Could you check a few things on this model? Use its own coordinates, in mm. Face numbers are marked on the shaded views. A direction names the side the tool comes from. Round coordinates to 2 decimals unless told otherwise and drop trailing zeros. Loops run counter-clockwise (first coordinate to the right, second up) from the corner with the lowest first, then second, coordinate; pieces in that order, holes last. Notation, with made-up numbers: (-26, -19) -> (-2, -19) arc R18 cw to (-2, 8) -> close; hole circle Ø4 at (25.5, 64). An arc over 180 degrees is marked (long way). One line per item, written item: value.
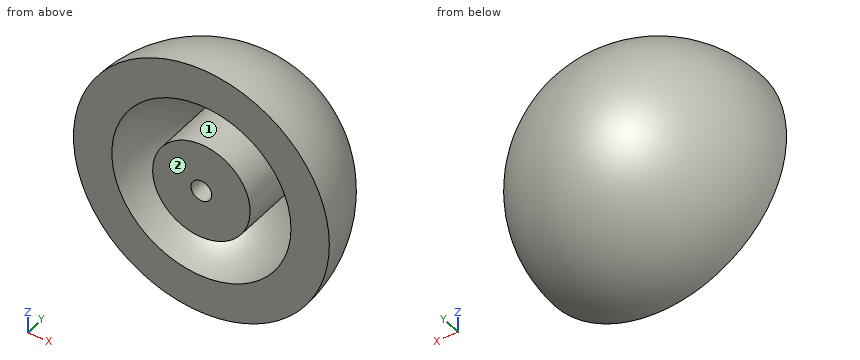
Autodesk Inventor part; units mm, degrees
ref_plane "YZ Plane" through (0, 0, 0) normal (1, 0, 0) x (0, 1, 0)
ref_plane "XZ Plane" through (0, 0, 0) normal (0, 1, 0) x (-1, 0, 0)
ref_plane "XY Plane" through (0, 0, 0) normal (0, 0, 1) x (1, 0, 0)
sketch "Sketch1" plane through (0, 0, 0) normal (0, 0, 1) x (1, 0, 0)
  line L0 (0, 0) -> (0, 20)
  line L1 (0, 0) -> (20, 0)
  arc A0 (20, 0) -> (0, 20) centre (0, 0) ccw
  line L2 (0, -4.8284) -> (0, 28.9706)
  dimension "d2" = 20
revolve "Revolution1" add sketch "Sketch1" angle 360 about axis through (0, -10, 0) along (0, 1, 0)
sketch "Sketch4" plane through (0, 0, 0) normal (0, -1, 0) x (1, 0, 0)
  point P0 (0, 0)
  point P1 (0, 0)
hole "Hole2" at (0, 0, 0) direction (0, 1, 0) diameter 3.242 depth 11.8 tip angle 118
shell "Shell2" thickness 6 removed faces 1 at (13.676, 0, 1.6606)
properties part number "Ball_Upper Half" material "Nylon 6/6"
Item 1: Will these pins go through, and if not, where does the flat tip stop? pin 1 Ø10 at (y, z) = (5, 3) entering from +X; pin 2 Ø5 at (x, y) = (15, 9.5) entering from +Z; pin 3 Ø10 at (y, z) = (14, -13) entering from +X.
Output:
pin 1: stops at x = 19.98
pin 2: stops at z = 12.93
pin 3: stops at x = 14.18
Item 2: If we section it at A-A on y = 8.25: List the corners of the cut face in (x, z) for me, plus the area to 3 significant figures.
Output:
outline: circle Ø36.44 at (0, 0); circle Ø15.24 at (0, 0); hole circle Ø22.62 at (0, 0); hole circle Ø3.24 at (0, 0)
area: 815 mm²
Item 3: If we section it at B-B on z = -3: List the corners of the cut face in (x, y) for me, plus the area to 3 significant figures.
Output:
outline: (-19.77, 0) -> (-13.67, 0) arc R13.67 cw to (-7.01, 11.74) -> (-7.01, 0) -> (7.01, 0) -> (7.01, 11.74) arc R13.67 cw to (13.67, 0) -> (19.77, 0) arc R19.77 ccw to start
area: 503 mm²
Item 4: I need wall thicknesses on line 1 (X direction, y = 6.75, z = 0); line 2 (Z direction, x = 0, y = 6); line 3 (Z direction, x = 0, y = 7.75). Which ranges of each line are inside material? Lowest first, please. Write a range as from..to.
Output:
line 1: x = -18.83..-12.27, -7.62..-1.62, 1.62..7.62, 12.27..18.83
line 2: z = -19.08..-12.65, -7.62..-1.62, 1.62..7.62, 12.65..19.08
line 3: z = -18.44..-11.66, -7.62..-1.62, 1.62..7.62, 11.66..18.44
Item 5: For the marked faces 1 and 2, which set-ups out of +Z, -Z, +X, -X, +Y, -Y let a thin tool reach every point of the face, with its end or its side?
Output:
face 1: -Y
face 2: +Z, -Z, +X, -X, -Y
Item 6: If we section it at D-D on x = -16: List the corners of the cut face in (y, z) for me.
Output:
outline: (0, -12) arc R12 ccw to (0, 12) -> close
Item 7: If we section it at C-C on x = -5: List the corners of the cut face in (y, z) for me.
Output:
outline: (0, -19.36) arc R19.36 ccw to (0, 19.36) -> (0, 13.08) arc R13.08 cw to (11.74, 5.75) -> (0, 5.75) -> (0, -5.75) -> (11.74, -5.75) arc R13.08 cw to (0, -13.08) -> close
